Geometry check sheet. Reference: the model listing, model coordinates, mm. Face numbers are marked on the shaded views. A direction names the side the tool comes from. Give positions to 0.01 mm unless a question says otherwise; leave off trailing zeros. Write each loop counter-clockwise with the first axis right and the second up, starting at its lowest first coordinate (ties: lowest second). Pieces come first, ordered by that corner, then holes.
(1) Mould release check, pull along Z, two halves, no side actions. Record for the marked faces 1, 2 and 3: +Z half, -Z half, draft (parallel to the pull), parting line (faces both ways), or undercut.
(2) Cross-section at B-B (z = 3.75). Record the boundary of the cut face in (x, y), and give its area (3 significant figures).
(3) Thickness scan on line 1 along Z through (x, y) = (-8.5, -1.75); line 2 along X through (y, z) = (7.5, 1); line 3 along X through (y, z) = (1, 2.25). Record the ranges inside material, lowest first.
(4) Cross-section at A-A (z = 2.5). Record the boundary of the cut face in (x, y).
(5) Depth check by flat-ended pin: P1, Ø0.6, axis at x = 0, y = 0, coming from the -Z side; P2, Ø1, axis at x = -7.5, z = 3.5, coming from the +Y side; P3, Ø1.5, axis at x = 0.5, y = -7, coming from the +Z side; P4, Ø1, axis at x = -0.5, y = -2, coming from the -Z side. Enter the tip coordinate at first touch or a pass-through.
(6) Tool access check on the marked faces 4 and 5. Record the directions out of +Z, -Z, +X, -X, +Y, -Y that give a thin tool (end or side, any length) a straight path to the whole face; none if there is none.
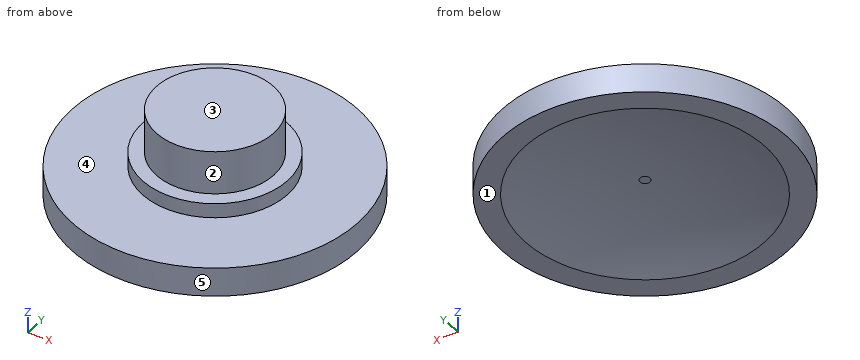
```python
from build123d import *

# Parameters (mm, degrees)
F0_R     = 9.8592181747
F1_DEPTH = 2
F2_R     = 5
F3_DEPTH = 1
F4_R     = 4.05
F5_DEPTH = 3
F6_R     = 8.2811029309
F7_DEPTH = 1


# Not quite as in the source:
# - a fillet or chamfer that OpenCascade refuses, or shapes differently, is made with other operations: its cross-section is extruded or revolved along the edge and cut away or added


with BuildPart() as f1:
    # F0 (on Top) → F1 (new body)
    with BuildSketch(Plane.XY):
        Circle(F0_R)
    extrude(amount=F1_DEPTH)

    # F2 (on face) → F3 (join)
    with BuildSketch(Plane.XY.offset(2)):
        Circle(F2_R)
    extrude(amount=F3_DEPTH)

    # F4 (on face) → F5 (join)
    with BuildSketch(Plane.XY.offset(3)):
        Circle(F4_R)
    extrude(amount=F5_DEPTH)

    # F6 (on face) → F7 (cut)
    with BuildSketch(Plane(origin=(0, 0, 0), x_dir=(1, 0, 0), z_dir=(0, 0, -1))):
        Circle(F6_R)
    extrude(amount=-F7_DEPTH, mode=Mode.SUBTRACT)

    # F8: fillet of radius 32 on 1 edges, made by hand

    # F8_s1 → F8_t2 (revolve)
    with BuildSketch(Plane.XZ):
        with BuildLine():
            ThreePointArc((8.2811029309, 0), (4.3438489977, 0.7490157328), (0.3438489977, 1))
            Line((0.3438489977, 1), (8.2811029309, 1))
            Line((8.2811029309, 1), (8.2811029309, 0))
        make_face()
    revolve(axis=Axis((0, 0, 1), (0, 0, -1)))


solid = f1.part
```
Reply:
1. face 1: -Z half
1. face 2: draft
1. face 3: +Z half
2. outline: circle Ø8.1 at (0, 0)
2. area: 51.5 mm2
3. line 1: z = 0 to 2
3. line 2: x = -6.4 to 6.4
3. line 3: x = -4.9 to 4.9
4. outline: circle Ø10 at (0, 0)
5. P1: stops at z = 1
5. P2: passes through
5. P3: stops at z = 2
5. P4: stops at z = 0.92
6. face 4: +Z
6. face 5: +Z, -Z
